For this review, take the finished solid that the model builds, in its own axes (mm). A direction names the side the tool comes from. Round coordinates to 2 decimals unless told otherwise and drop trailing zeros. Loops run counter-clockwise (first coordinate to the right, second up) from the corner with the lowest first, then second, coordinate; pieces in that order, holes last. Notation, with made-up numbers: M -33.5,59.5 L 6.5,59.5 A17 ccw 6.5,66.5 Z; hole C 45.5,15 d3. An arc over 180 degrees is marked long. One line per question, with ' | ' between items. Start each with the question number.
1) We need section A-A (x = 6). Give the boundary of the cut face in (y, z).
2) For probe 1 along Y at (x, z) = (-15, 3.7); probe 2 along X at (y, z) = (-10.75, 2.7); probe 3 along Y at (x, z) = (-2, 0.45), list the stretches that pass through material, from the lowest coordinate up. Write a range as from..to.
3) Mouldability with a two-part tool opening along Y and no side actions: class faces 1 (the face through (1, -3, 0)), 2 (the face through (0.57, -24.4, 2.54)), 3 (the face through (10, -12, 2)) as pulls with the +Y half, pulls with the -Y half, needs draft (parallel to the pull), parting line crosses it, or undercut.
4) For faces 4 (the face through (0, -22.5, 2.5)), 5 (the face through (5, -20, 2)), 6 (the face through (14.4, 4.43, 2.54)), list the 3-axis set-ups (+Z, -Z, +X, -X, +Y, -Y) from which the entire face can be reached by the end or side of a thin tool; tool diameter is ignored.
5) We need section D-D (y = -14). Give the boundary of the cut face in (x, z), and give its area (3 significant figures).
6) We need section B-B (y = 0). Give the boundary of the cut face in (x, z).
7) We need section C-C (z = 3.3). Give the boundary of the cut face in (x, y), and give its area (3 significant figures).
8) For pin 1 Ø0.8 at (y, z) = (-22.5, 3.5) entering from -X, flat-tipped, find the tip position at first contact; note if it passes through.
```python
from build123d import *

# Parameters (mm, degrees)
ESQUISSE1_R        = 2.5
BOSS_EXTRU_1_DEPTH = 5
CONG_1_R           = 2


with BuildPart() as part:
    # Esquisse1 → Boss.-Extru.1 (new body)
    with BuildSketch(Plane.XY):
        with BuildLine():
            Line((10, -5), (10, -20))
            Line((10, -20), (0, -20))
            Line((0, -20), (0, -25))
            Line((0, -25), (15, -25))
            Line((15, -25), (15, -5))
            Line((15, -5), (15, 5))
            Line((15, 5), (-15, 5))
            ThreePointArc((-15, 5), (-20, 0), (-15, -5))
            Line((-15, -5), (10, -5))
        make_face()
        with Locations((-15, 0)):
            Circle(ESQUISSE1_R, mode=Mode.SUBTRACT)
    extrude(amount=BOSS_EXTRU_1_DEPTH)

    # Congé1
    cong_1_edges = [part.edges().sort_by_distance(p)[0] for p in [
        (15, -25, 2.5),
        (0, -25, 2.5),
        (0, -20, 2.5),
        (10, -20, 2.5),
        (10, -5, 2.5),
        (15, 5, 2.5),
    ]]
    fillet(cong_1_edges, radius=CONG_1_R)


solid = part.part
```
Answers below:
1) outline: M -25,0 L -20,0 L -20,5 L -25,5 Z; M -5,0 L 5,0 L 5,5 L -5,5 Z
2) probe 1: -5..-2.5, 2.5..5 | probe 2: 10..15 | probe 3: -5..5
3) face 1: needs draft | face 2: pulls with the -Y half | face 3: undercut
4) face 4: +Z, -Z, -X, -Y | face 5: +Z, -Z, -X | face 6: +Z, -Z, +X, +Y
5) outline: M 10,0 L 15,0 L 15,5 L 10,5 Z | area: 25.0 mm^2
6) outline: M -20,0 L -17.5,0 L -17.5,5 L -20,5 Z; M -12.5,0 L 15,0 L 15,5 L -12.5,5 Z
7) outline: M -15,-5 L 8,-5 A2 cw 10,-7 L 10,-18 A2 cw 8,-20 L 2,-20 A2 ccw 0,-22 L 0,-23 A2 ccw 2,-25 L 13,-25 A2 ccw 15,-23 L 15,3 A2 ccw 13,5 L -15,5 A5 ccw Z; hole C -15,0 d5 | area: 468 mm^2
8) pin 1: x = 0
